```python
from build123d import *

# Parameters (mm, degrees)
F0_W      = 304.8
F0_H      = 38.1
F1_DEPTH  = 19.05
F2_R      = 11.1125
F3_DEPTH  = 12.7
F4_R      = 3.175
F5_DEPTH  = 19.051
F6_R      = 3.175
F7_DEPTH  = 19.051
F8_R      = 0.79375
F9_DEPTH  = 19.051
F10_W     = 3.175
F10_H     = 1.5875
F11_DEPTH = 38.101


with BuildPart() as f1:
    # F0 (on Top) → F1 (new body)
    with BuildSketch(Plane.XY):
        with Locations((84.480461, 0)):
            Rectangle(F0_W, F0_H)
    extrude(amount=F1_DEPTH)

    # F2 (on face) → F3 (cut)
    with BuildSketch(Plane.XY.offset(19.05)):
        with Locations((135.280461, 0)):
            Circle(F2_R)
    extrude(amount=-F3_DEPTH, mode=Mode.SUBTRACT)

    # F4 (on face) → F5 (cut, through all)
    with BuildSketch(Plane.XY.offset(19.05)):
        with Locations((-58.394539, -3.175)):
            Circle(F4_R)
    extrude(amount=-F5_DEPTH, mode=Mode.SUBTRACT)

    # F6 (on face) → F7 (cut, through all)
    with BuildSketch(Plane.XY.offset(19.05)):
        with Locations((-24.612539, -9.525)):
            Circle(F6_R)
        with Locations((-24.612539, 9.525)):
            Circle(F6_R)
    extrude(amount=-F7_DEPTH, mode=Mode.SUBTRACT)

    # F8 (on face) → F9 (cut, through all)
    with BuildSketch(Plane.XY.offset(19.05)):
        with Locations((230.530461, 9.525)):
            Circle(F8_R)
        with Locations((230.530461, 0)):
            Circle(F8_R)
        with Locations((230.530461, -9.525)):
            Circle(F8_R)
    extrude(amount=-F9_DEPTH, mode=Mode.SUBTRACT)

    # F10 (on face) → F11 (cut, through all)
    with BuildSketch(Plane.XZ.offset(19.05)):
        with Locations((-9.182039, 18.25625)):
            Rectangle(F10_W, F10_H)
        with Locations((216.242961, 18.25625)):
            Rectangle(F10_W, F10_H)
    extrude(amount=-F11_DEPTH, mode=Mode.SUBTRACT)


solid = f1.part
```
The listing builds one solid part. Answer for the finished solid, in the listing's coordinates (mm). A direction names the side the tool comes from. Round coordinates to 2 decimals unless told otherwise and drop trailing zeros. Use one line per item in the form item = value.
1. A tool of negligible diameter and unlimited length cuts with its end or side. For faces 5 (the flat face through (135, 0, 6.35)), 6 (the flat face through (227, 0, 19.05)), from which of +Z, -Z, +X, -X, +Y, -Y can it reach the whole face along a straight path? Write none if from no direction.
Answer key:
face_5 = +Z
face_6 = +Z, +X, -X, +Y, -Y
2. For a pull along Y with two mould halves and no side action, classify faces 1 (the flat face through (82, 0, 0)), 2 (the flat face through (82, -19.05, 9)), 3 (the cylindrical face through (-21.68, -10.74, 9.66)), 4 (the cylindrical face through (-21.584, 10.479, 9.658)) as released by +Y, released by -Y, zero draft, split by the parting line, or undercut.
Answer key:
face_1 = zero draft
face_2 = released by -Y
face_3 = undercut
face_4 = undercut
3. Flat-ended cylindrical pins translate along their axes: pin 1 Ø1.6 at (x, y) = (-8.5, -9) entering from +Z; pin 2 Ø6.5 at (x, y) = (132, -1) entering from +Z; pin 3 Ø1 at (x, y) = (230.53, 0) entering from +Z. Find the tip coordinate at first contact, or state that the pin passes through.
Answer key:
pin_1 = 17.46
pin_2 = 6.35
pin_3 = through
4. The part is cut by section A-A on z = 10.5. Give the number of separate pieces and of enclosed holes in the cut face, and give its area (3 significant figures).
Answer key:
separate_pieces = 1
enclosed_holes = 7
area = 11,100 mm²
5. Find the intervals of material crossed by probe 1 along X at (y, z) = (9.5, 14.75); probe 2 along X at (y, z) = (1, 7.75); probe 3 along X at (y, z) = (-1, 17), in increasing order. Write a range as [from, to].
Answer key:
probe_1 = [-67.92, -27.79], [-21.44, 129.52], [141.05, 229.74], [231.32, 236.88]
probe_2 = [-67.92, 124.21], [146.35, 236.88]
probe_3 = [-67.92, -60.71], [-56.08, 124.21], [146.35, 236.88]
